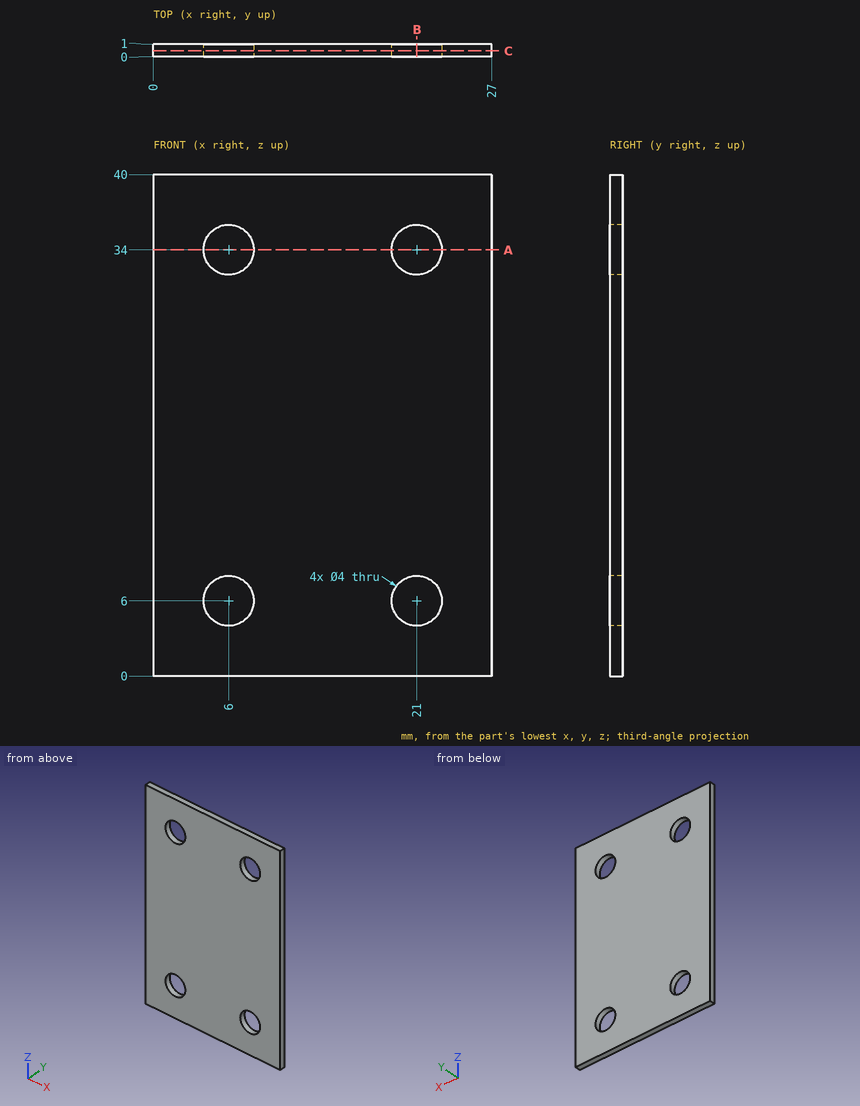
The drawing under review shows one solid part. Ordinate dimensions are in mm from its lowest x, y, z. Give positions to 0.01 mm unless a question says otherwise; leave off trailing zeros. Loops run counter-clockwise (first coordinate to the right, second up) from the corner with the lowest first, then second, coordinate; pieces in that order, holes last. Notation, with made-up numbers: M 19.25,9 L 53.25,9 A17 ccw 53.25,18 Z; hole C 59,36.25 d6. An arc over 180 degrees is marked long. Return JSON: item names as keys, results as strings. Group by question number.
Item 1: We need section B-B (x = 21). Give the boundary of the cut face in (y, z), and give its area (3 significant figures).
Item 2: Insertion check: pin 1 Ø3.5 at (x, z) = (6, 34) entering from +Y. The pin has a flat end and moves straight along its axis. Give the tip position at first contact, or say it passes through.
Item 3: For probe 1 along Z at (x, y) = (6, 0.45); probe 2 along Z at (x, y) = (4.75, 0.7), list the stretches that pass through material, from the lowest coordinate up.
Item 4: We need section C-C (y = 0.45). Give the boundary of the cut face in (x, z), and give its area (3 significant figures).
Item 5: We need section A-A (z = 34). Give the boundary of the cut face in (x, y).
Output:
{
 "1": {"outline": "M 0,0 L 1,0 L 1,4 L 0,4 Z; M 0,8 L 1,8 L 1,32 L 0,32 Z; M 0,36 L 1,36 L 1,40 L 0,40 Z", "area": "32.0 mm^2"},
 "2": {"pin 1": "passes through"},
 "3": {"probe 1": "z = 0 to 4, 8 to 32, 36 to 40", "probe 2": "z = 0 to 4.44, 7.56 to 32.44, 35.56 to 40"},
 "4": {"outline": "M 0,0 L 27,0 L 27,40 L 0,40 Z; hole C 6,6 d4; hole C 6,34 d4; hole C 21,6 d4; hole C 21,34 d4", "area": "1,030 mm^2"},
 "5": {"outline": "M 0,0 L 4,0 L 4,1 L 0,1 Z; M 8,0 L 19,0 L 19,1 L 8,1 Z; M 23,0 L 27,0 L 27,1 L 23,1 Z"}
}
